Geometry: see drawing. Coordinates: mm, zero at the bounding-box minimum. A direction names the side the tool comes from. Give positions to 0.01 mm unless a question says otherwise; leave off trailing zeros. Order: outer loops, then holes, each group sorted by start corner. A loop starts at its lowest first (then second) coordinate and runs counter-clockwise, first axis right, second up. Notation, with made-up numbers: M 52,21 L 104,21 A32 ccw 104,60 Z; hole C 54.25,48.5 d1. An arc over 180 degrees is marked long. Write item = value, one per line. Start each with the question number.
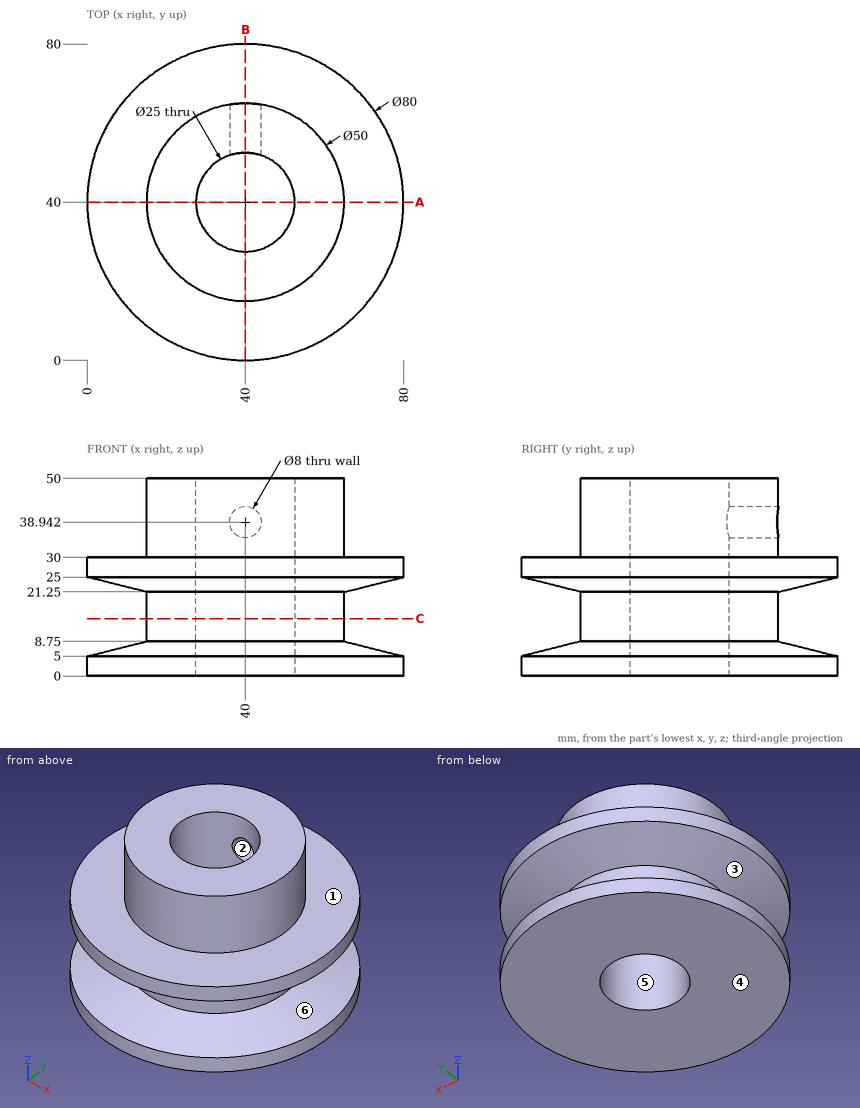
1) Access query for the marked faces 1, 2 and 3. Directions: +Z, -Z, +X, -X, +Y, -Y. A direction counts if a zero-diameter tool reaches every point of the face in a straight line with its end or side. Return the directions, or none.
2) Cut plane C-C (z = 14.5). Return loops of the section in (x, y), plus the area to 3 significant figures.
3) Draft query along X for the marked faces 4, 5 and 6. Return one class per face: pulls with the +X half, pulls with the -X half, needs draft (parallel to the pull), parting line crosses it, or undercut.
4) Cut plane B-B (x = 40). Return loops of the section in (y, z), plus the area to 3 significant figures.
5) Ray query, L1, parallel to Y at x = 40, z = 20; L2, parallel to Z at x = 40, y = 56; L3, parallel to Y at x = 29.5, z = 40. Return the intervals inside material, ascending.
6) Cut plane A-A (y = 40). Return loops of the section in (x, z).
7) Pin query (flat end, axial travel): pin 1 Ø1.5 at (x, y) = (36.5, 49.5) entering from +Z; pin 2 Ø10 at (x, y) = (13.5, 17) entering from +Z; pin 3 Ø9 at (x, z) = (40, 38.94) entering from -Y; pin 4 Ø6 at (y, z) = (61, 28) entering from +X. Return the tip coordinate at first contact, or that it passes through.
Reply:
q1.face_1 = +Z
q1.face_2 = +Y
q1.face_3 = none
q2.outline = C 40,40 d50; hole C 40,40 d25
q2.area = 1,470 mm²
q3.face_4 = needs draft
q3.face_5 = undercut
q3.face_6 = parting line crosses it
q4.outline = M 0,0 L 27.5,0 L 27.5,50 L 15,50 L 15,30 L 0,30 L 0,25 L 15,21.25 L 15,8.75 L 0,5 Z; M 52.5,0 L 80,0 L 80,5 L 65,8.75 L 65,21.25 L 80,25 L 80,30 L 65,30 L 65,34.94 L 52.5,34.94 Z; M 52.5,42.94 L 65,42.94 L 65,50 L 52.5,50 Z
q4.area = 1,560 mm²
q5.L1 = 15 to 27.5, 52.5 to 65
q5.L2 = 0 to 34.94, 42.94 to 50
q5.L3 = 17.31 to 33.22, 46.78 to 62.69
q6.outline = M 0,0 L 27.5,0 L 27.5,50 L 15,50 L 15,30 L 0,30 L 0,25 L 15,21.25 L 15,8.75 L 0,5 Z; M 52.5,0 L 80,0 L 80,5 L 65,8.75 L 65,21.25 L 80,25 L 80,30 L 65,30 L 65,50 L 52.5,50 Z
q7.pin_1 = through
q7.pin_2 = 30
q7.pin_3 = 15
q7.pin_4 = 75.72
